from build123d import *

# Parameters (mm, degrees)
BOSS_EXTRUDE1_DEPTH = 500
FILLET1_R           = 6
FILLET2_R           = 3
SKETCH2_W           = 10
SKETCH2_H           = 3
SKETCH2_W_2         = 6
SKETCH2_W_3         = 6.201832359
SKETCH2_W_4         = 3
SKETCH2_H_2         = 8
CUT_EXTRUDE1_DEPTH  = 50


with BuildPart() as part:
    # Sketch1 → Boss-Extrude1 (new body, symmetric)
    with BuildSketch(Plane.XY):
        Polygon((0, 0), (30, 0), (30, 50), (0, 50), (0, 35), (3, 35), (3, 47), (27, 47), (27, 3), (3, 3), (3, 15), (0, 15), align=None)
    extrude(amount=BOSS_EXTRUDE1_DEPTH, both=True)

    # Fillet1
    fillet1_edges = [part.edges().sort_by_distance(p)[0] for p in [
        (0, 50, 0),
        (30, 50, 0),
        (30, 0, 0),
        (0, 0, 0),
    ]]
    fillet(fillet1_edges, radius=FILLET1_R)

    # Fillet2
    fillet2_edges = [part.edges().sort_by_distance(p)[0] for p in [
        (3, 3, 0),
        (27, 3, 0),
        (27, 47, 0),
        (3, 47, 0),
    ]]
    fillet(fillet2_edges, radius=FILLET2_R)

    # Sketch2 → Cut-Extrude1 (cut)
    with BuildSketch(Plane(origin=(0, 50, 0), x_dir=(1, 0, 0), z_dir=(0, 1, 0))):
        with Locations((15, 498.5)):
            Rectangle(SKETCH2_W, SKETCH2_H)
        with Locations((3, 498.5)):
            Rectangle(SKETCH2_W_2, SKETCH2_H)
        with Locations((3, -498.5)):
            Rectangle(SKETCH2_W_2, SKETCH2_H)
        with Locations((15, -498.5)):
            Rectangle(SKETCH2_W, SKETCH2_H)
        with Locations((14.859499195, 490.5)):
            Rectangle(SKETCH2_W_3, SKETCH2_H)
        with Locations((14.859499195, 473.5)):
            Rectangle(SKETCH2_W_3, SKETCH2_H)
        with Locations((21, 482)):
            Rectangle(SKETCH2_W_4, SKETCH2_H_2)
        with Locations((14.859499195, -473.5)):
            Rectangle(SKETCH2_W_3, SKETCH2_H)
        with Locations((21, -482)):
            Rectangle(SKETCH2_W_4, SKETCH2_H_2)
        with Locations((14.859499195, -490.5)):
            Rectangle(SKETCH2_W_3, SKETCH2_H)
    extrude(amount=-CUT_EXTRUDE1_DEPTH, mode=Mode.SUBTRACT)


solid = part.part
Check sheet for the modelled part. Datum: model origin and axes. Units: mm. A direction names the side the tool comes from. Give positions to 0.01 mm unless a question says otherwise; leave off trailing zeros. Write each loop counter-clockwise with the first axis right and the second up, starting at its lowest first coordinate (ties: lowest second). Pieces come first, ordered by that corner, then holes. Notation, with made-up numbers: (-33.75, -35) -> (24.25, -35) arc R22 ccw to (24.25, -28) -> close; hole circle Ø7 at (19, 41). An arc over 180 degrees is marked (long way). Use one line per item in the form item = value. Start each with the question number.
1. Go/stop test with flat-tipped pins: P1, Ø6, axis at x = 18, y = 5.5, coming from the +Z side; P2, Ø3.5, axis at x = 13.5, y = 48, coming from the -Z side; P3, Ø10, axis at x = 19, z = -135.5, coming from the -Y side; P4, Ø0.9, axis at y = 2, z = -491, coming from the -X side. Record where each tip stops, or that it passes through.
2. Mould release check, pull along Y, two halves, no side actions. Record for faces 1 (the flat face through (30, 25, 7)), 2 (the flat face through (15, 3, 7)), 3 (the flat face through (15, 0, 7)), 4 (the flat face through (27, 25, 7)): pulls with the +Y half, pulls with the -Y half, needs draft (parallel to the pull), parting line crosses it, or undercut.
3. Section check A-A (z = 30.5). Record the cut outline in (x, y).
4. Thickness scan on line 1 along X through (y, z) = (8.5, -38); line 2 along Y through (x, z) = (10.25, -290.5); line 3 along X through (y, z) = (19.5, -359). Record the ranges inside material, lowest first. Write a range as from..to.
5. Access from +Z, -Z, +X, -X, +Y, -Y to the whole of each face (thin tool, end or side, straight path). Record for faces 5 (the flat face through (15, 50, 7)), 6 (the flat face through (15, 47, 7)).
Conclusion:
q1.P1 = 497
q1.P2 = -497
q1.P3 = 0
q1.P4 = 1.16
q2.face_1 = needs draft
q2.face_2 = undercut
q2.face_3 = pulls with the -Y half
q2.face_4 = undercut
q3.outline = (0, 6) arc R6 ccw to (6, 0) -> (24, 0) arc R6 ccw to (30, 6) -> (30, 44) arc R6 ccw to (24, 50) -> (6, 50) arc R6 ccw to (0, 44) -> (0, 35) -> (3, 35) -> (3, 44) arc R3 cw to (6, 47) -> (24, 47) arc R3 cw to (27, 44) -> (27, 6) arc R3 cw to (24, 3) -> (6, 3) arc R3 cw to (3, 6) -> (3, 15) -> (0, 15) -> close
q4.line_1 = 0..3, 27..30
q4.line_2 = 0..3, 47..50
q4.line_3 = 27..30
q5.face_5 = +Z, -Z, +X, -X, +Y
q5.face_6 = +Z, -Z
